```python
from build123d import *

# Parameters (mm, degrees)
SKETCH_R  = 1.55
PAD_DEPTH = 3


with BuildPart() as part:
    # Sketch → Pad (new body)
    with BuildSketch(Plane.XY):
        with BuildLine():
            Line((83.5225, 17.4775), (301.2275, 17.4775))
            ThreePointArc((303.2275, 15.4775), (302.641714, 16.891714), (301.2275, 17.4775))
            Line((303.2275, 15.4775), (303.2275, -91.6775))
            ThreePointArc((301.2275, -93.6775), (302.641714, -93.091714), (303.2275, -91.6775))
            Line((301.2275, -93.6775), (-15.4775, -93.6775))
            ThreePointArc((-17.4775, -91.6775), (-16.891714, -93.091714), (-15.4775, -93.6775))
            Line((-17.4775, -91.6775), (-17.4775, -43.006))
            Line((-17.4775, -43.006), (-10.3335, -43.006))
            Line((-10.3335, -43.006), (-10.3335, -86.5335))
            Line((-10.3335, -86.5335), (296.0835, -86.5335))
            Line((296.0835, 10.3335), (296.0835, -86.5335))
            Line((83.5225, 10.3335), (296.0835, 10.3335))
            Line((83.5225, 17.4775), (83.5225, 10.3335))
        make_face()
        with Locations((-13.9055, -90.1055)):
            Circle(SKETCH_R, mode=Mode.SUBTRACT)
        with Locations((195.135167, -90.1055)):
            Circle(SKETCH_R, mode=Mode.SUBTRACT)
        with Locations((299.6555, -90.1055)):
            Circle(SKETCH_R, mode=Mode.SUBTRACT)
        with Locations((90.614833, -90.1055)):
            Circle(SKETCH_R, mode=Mode.SUBTRACT)
        with Locations((90.614833, 13.9055)):
            Circle(SKETCH_R, mode=Mode.SUBTRACT)
        with Locations((195.135167, 13.9055)):
            Circle(SKETCH_R, mode=Mode.SUBTRACT)
        with Locations((299.6555, 13.9055)):
            Circle(SKETCH_R, mode=Mode.SUBTRACT)
        with Locations((-13.9055, -46.578)):
            Circle(SKETCH_R, mode=Mode.SUBTRACT)
    extrude(amount=PAD_DEPTH)


solid = part.part
```
Source: CAD feature listing. Evaluate the final solid. Frame: model axes, mm. Give positions to 0.01 mm unless a question says otherwise; leave off trailing zeros. Order: outer loops, then holes, each group sorted by start corner. A loop starts at its lowest first (then second) coordinate and runs counter-clockwise, first axis right, second up.
(1) Section query C-C (z = 0.45). State how many separate pieces and enclosed holes the cut face has, plus the area to 3 significant figures.
(2) Section query B-B (y = -51.5). Return the cut outline in (x, z), plus the area to 3 significant figures.
(3) Section query D-D (x = 61.5). Return the cut outline in (y, z), plus the area to 3 significant figures.
(4) Section query A-A (x = 190). Return the cut outline in (y, z).
(5) Contact query for flat-ended pins moving along their axis: P1, Ø0.9, axis at x = -15, z = 1, coming from the +Y side; P2, Ø0.9, axis at y = 15, z = 1.5, coming from the -X side; P3, Ø3.5, axis at x = -13.91, y = -46.58, coming from the +Z side. Output: stop coordinate, or through.
(6) Material intervals for line 1 along X through (y, z) = (-77.5, 1.15); line 2 along Y through (x, z) = (271, 1); line 3 along X through (y, z) = (-47.5, 1.8), sorted ascending.
Outcome:
1. separate pieces: 1
1. enclosed holes: 8
1. area: 4,800 mm2
2. outline: (-17.48, 0) - (-10.33, 0) - (-10.33, 3) - (-17.48, 3) - close; (296.08, 0) - (303.23, 0) - (303.23, 3) - (296.08, 3) - close
2. area: 42.9 mm2
3. outline: (-93.68, 0) - (-86.53, 0) - (-86.53, 3) - (-93.68, 3) - close
3. area: 21.4 mm2
4. outline: (-93.68, 0) - (-86.53, 0) - (-86.53, 3) - (-93.68, 3) - close; (10.33, 0) - (17.48, 0) - (17.48, 3) - (10.33, 3) - close
5. P1: stops at y = -43.01
5. P2: stops at x = 83.52
5. P3: stops at z = 3
6. line 1: x = -17.48 to -10.33, 296.08 to 303.23
6. line 2: y = -93.68 to -86.53, 10.33 to 17.48
6. line 3: x = -17.48 to -15.15, -12.66 to -10.33, 296.08 to 303.23
